from build123d import *

# Parameters (mm, degrees)
SKETCH1_R           = 0.3207
SKETCH1_W           = 0.5
SKETCH1_H           = 1.6
BOSS_EXTRUDE1_DEPTH = 0.5
SKETCH1_24_W        = 0.5
SKETCH1_24_H        = 1.6
BOSS_EXTRUDE2_DEPTH = 3


with BuildPart() as part:
    # Sketch1 → Boss-Extrude1 (new body)
    # profile 1 of 4: a face of its own
    with BuildSketch(Plane(origin=(0, 0, 0), x_dir=(1, 0, 0), z_dir=(0, 1, 0))):
        with BuildLine():
            ThreePointArc((0.1641009, 1.993256355), (0.024548565, 1.994973575), (-0.113883759, 1.977245221))
            Line((-0.113883759, 1.977245221), (-1.25, 1.750241174))
            Line((-1.25, 1.750241174), (-1.25, 1.25))
            ThreePointArc((-1.25, 1.25), (-0.366116524, 0.883883476), (0, 0))
            ThreePointArc((0, 0), (-0.366116524, -0.883883476), (-1.25, -1.25))
            Line((-1.25, -1.25), (-1.25, -1.750241174))
            Line((-1.25, -1.750241174), (-0.11388376, -1.977245221))
            ThreePointArc((-0.11388376, -1.977245221), (0.024548564, -1.994973575), (0.164100898, -1.993256355))
            ThreePointArc((0.164100898, -1.993256355), (2, -1e-09), (0.1641009, 1.993256355))
        make_face()
        with Locations(Location((0.5, 0, 0), (0, 0, 270))):
            Circle(SKETCH1_R, mode=Mode.SUBTRACT)
        with BuildLine():
            Line((0, 1.3), (0, 1.6))
            ThreePointArc((0, 1.6), (1.6, 0), (0, -1.6))
            Line((0, -1.6), (0, -1.3))
            ThreePointArc((0, -1.3), (1.3, 0), (0, 1.3))
        make_face(mode=Mode.SUBTRACT)
    # profile 2 of 4: a face of its own
    with BuildSketch(Plane(origin=(0, 0, 0), x_dir=(1, 0, 0), z_dir=(0, 1, 0))):
        with BuildLine():
            Line((-1.25, 1.25), (-1.25, 1.750241174))
            Line((-1.25, 1.750241174), (-4.183235691, 1.164159973))
            ThreePointArc((-4.183235691, 1.164159973), (-4.514100231, 1.033532975), (-4.77830642, 0.795352694))
            ThreePointArc((-4.77830642, 0.795352694), (-5.05, 0), (-4.77830642, -0.795352694))
            ThreePointArc((-4.77830642, -0.795352694), (-4.514100231, -1.033532975), (-4.183235691, -1.164159973))
            Line((-4.183235691, -1.164159973), (-1.25, -1.750241174))
            Line((-1.25, -1.750241174), (-1.25, -1.25))
            ThreePointArc((-1.25, -1.25), (-2.5, 0), (-1.25, 1.25))
        make_face()
        with Locations((-4, 0)):
            Rectangle(SKETCH1_W, SKETCH1_H, mode=Mode.SUBTRACT)
        with Locations(Location((-3, 0, 0), (0, 0, 270))):
            Circle(SKETCH1_R, mode=Mode.SUBTRACT)
    # profile 3 of 4: a face of its own
    with BuildSketch(Plane(origin=(0, 0, 0), x_dir=(1, 0, 0), z_dir=(0, 1, 0))):
        with BuildLine():
            Line((0, 1.6), (0, 1.3))
            ThreePointArc((0, 1.3), (1.3, 0), (0, -1.3))
            Line((0, -1.3), (0, -1.6))
            ThreePointArc((0, -1.6), (1.6, 0), (0, 1.6))
        make_face()
    # profile 4 of 4: a face of its own
    with BuildSketch(Plane(origin=(0, 0, 0), x_dir=(1, 0, 0), z_dir=(0, 1, 0))):
        with Locations((-4, 0)):
            Rectangle(SKETCH1_W, SKETCH1_H)
    extrude(amount=BOSS_EXTRUDE1_DEPTH)

    # Sketch1_24 → Boss-Extrude2 (add)
    with BuildSketch(Plane(origin=(0, 0, 0), x_dir=(1, 0, 0), z_dir=(0, 1, 0))):
        with Locations((-4, 0)):
            Rectangle(SKETCH1_24_W, SKETCH1_24_H)
        with BuildLine():
            Line((0, 1.6), (0, 1.3))
            ThreePointArc((0, 1.3), (1.3, 0), (0, -1.3))
            Line((0, -1.3), (0, -1.6))
            ThreePointArc((0, -1.6), (1.6, 0), (0, 1.6))
        make_face()
    extrude(amount=BOSS_EXTRUDE2_DEPTH)


solid = part.part
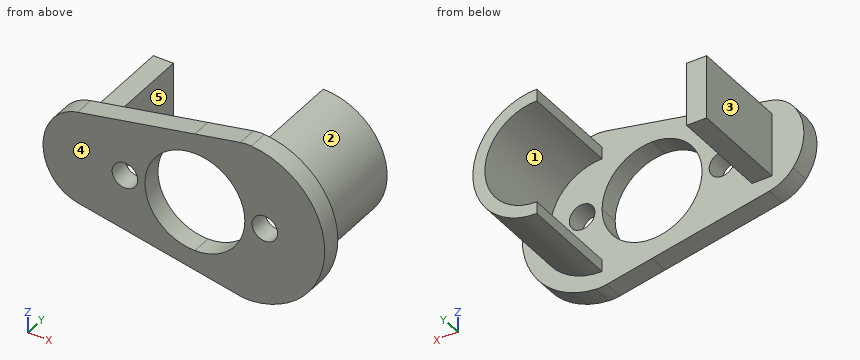
Geometry: final body of the model. Coordinates: model frame, mm. Face numbers are marked on the shaded views. A direction names the side the tool comes from. Coordinates: 2 decimals unless noted, no trailing zeros. Order: outer loops, then holes, each group sorted by start corner. A loop starts at its lowest first (then second) coordinate and runs counter-clockwise, first axis right, second up.
(1) Section query C-C (y = 0.3). Return the cut outline in (x, z).
(2) Section query A-A (y = 2.65). Return the cut outline in (x, z).
(3) First-contact query: pin 1 (1 mm diameter, centred on x = 0, z = -1, fed in from -Y); pin 2 (1 mm diameter, centred on y = 2, z = 0, fed in from -X); pin 3 (0.8 mm diameter, centred on y = 2, z = 0, fed in from +X). Flat tips, straight axial feed; report the tip coordinate or a pass-through.
(4) Section query B-B (x = 0.5). Return the cut outline in (y, z).
(5) Section query D-D (z = 0.55). Return the cut outline in (x, y), plus the area to 3 significant figures.
(6) Access query for the marked faces 4 and 5. Directions: +Z, -Z, +X, -X, +Y, -Y. A direction counts if a zero-diameter tool reaches every point of the face in a straight line with its end or side. Return the directions, or none.
(7) Draft query along Z for the marked faces 1, 2 and 3. Return one class per face: pulls with the +Z half, pulls with the -Z half, needs draft (parallel to the pull), parting line crosses it, or undercut.
(8) Material intervals for probe 1 along X at (y, z) = (0.4, -0.25); probe 2 along Y at (x, z) = (0.5, 1); probe 3 along Z at (x, y) = (0.25, 2.8), sorted ascending.
Solution:
1. outline: (-4.78, -0.8) arc R1 ccw to (-4.18, -1.16) - (-0.11, -1.98) arc R1 ccw to (0.16, -1.99) arc R2 ccw to (0.16, 1.99) arc R1 ccw to (-0.11, 1.98) - (-4.18, 1.16) arc R1 ccw to (-4.78, 0.8) arc R1.3 ccw to start; hole circle Ø0.64 at (-3, 0); hole circle Ø2.5 at (-1.25, 0); hole circle Ø0.64 at (0.5, 0)
2. outline: (-4.25, -0.8) - (-3.75, -0.8) - (-3.75, 0.8) - (-4.25, 0.8) - close; (0, -1.6) arc R1.6 ccw to (0, 1.6) - (0, 1.3) arc R1.3 cw to (0, -1.3) - close
3. pin 1: stops at y = 0
3. pin 2: stops at x = -4.25
3. pin 3: stops at x = 1.6
4. outline: (0, -1.94) - (0.5, -1.94) - (0.5, -1.52) - (3, -1.52) - (3, -1.2) - (0.5, -1.2) - (0.5, -0.32) - (0, -0.32) - close; (0, 0.32) - (0.5, 0.32) - (0.5, 1.2) - (3, 1.2) - (3, 1.52) - (0.5, 1.52) - (0.5, 1.94) - (0, 1.94) - close
5. outline: (-4.93, 0) - (-2.37, 0) - (-2.37, 0.5) - (-3.75, 0.5) - (-3.75, 3) - (-4.25, 3) - (-4.25, 0.5) - (-4.93, 0.5) - close; (-0.13, 0) - (1.92, 0) - (1.92, 0.5) - (1.5, 0.5) - (1.5, 3) - (1.18, 3) - (1.18, 0.5) - (-0.13, 0.5) - close
5. area: 4.36 mm2
6. face 4: +Z, -Z, +X, -X, -Y
6. face 5: +Z, -Z, +Y
7. face 1: undercut
7. face 2: parting line crosses it
7. face 3: needs draft
8. probe 1: x = -5.03 to -3.2, -2.8 to -2.47, -0.03 to 0.3, 0.7 to 1.98
8. probe 2: y = 0 to 0.5
8. probe 3: z = -1.58 to -1.28, 1.28 to 1.58
